Input: part model. Units: mm. Frame: model coordinates. Face numbers are marked on the shaded views. Coordinates: 2 decimals unless noted, no trailing zeros. Order: outer loops, then holes, each group sorted by start corner. A loop starts at its lowest first (then second) coordinate and runs counter-clockwise, first axis right, second up. Notation, with made-up numbers: (-23.75, 12) -> (28.25, 12) arc R15 cw to (28.25, 17) -> close; hole circle Ø4 at (52.5, -34). An arc over 180 degrees is marked (long way). One line per question, with ' | ' between items.
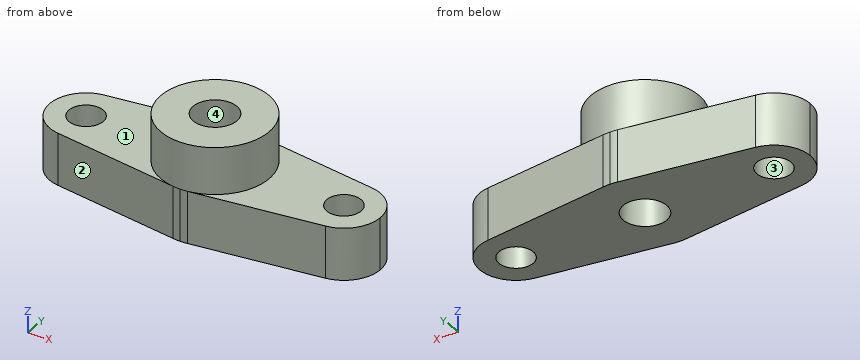
```python
from build123d import *

# Parameters (mm, degrees)
SKETCH_1_W             = 32
SKETCH_1_H             = 10.4
SKETCH_1_R             = 0.5
EXTRUDE_1_DEPTH        = 5
SKETCH_2_R             = 5.2
SKETCH_2_R_2           = 0.5
EXTRUDE_2_DEPTH        = 4.5
CUT_EXTRUDE_START      = -5.3
CUT_EXTRUDE_1_DEPTH    = 5.3
HOLE_WIZARD_M4_1_D     = 3.3
HOLE_WIZARD_M4_1_DEPTH = 10.1
HOLE_WIZARD_M4_1_TIP   = 0.991420021
HOLE_WIZARD_M5_1_D     = 4.2
HOLE_WIZARD_M5_1_DEPTH = 22.4
HOLE_WIZARD_M5_1_TIP   = 1.2618073


with BuildPart() as part:
    # 草图1 → 凸台-拉伸1 (new body)
    with BuildSketch(Plane.XY):
        Rectangle(SKETCH_1_W, SKETCH_1_H)
        with Locations((-12.5, 0)):
            Circle(SKETCH_1_R, mode=Mode.SUBTRACT)
        with Locations((12.5, 0)):
            Circle(SKETCH_1_R, mode=Mode.SUBTRACT)
        Circle(SKETCH_1_R, mode=Mode.SUBTRACT)
    extrude(amount=EXTRUDE_1_DEPTH)

    # 草图2 → 凸台-拉伸2 (add)
    with BuildSketch(Plane.XY.offset(5)):
        with Locations(Location((0, 0, 0), (0, 0, 270))):
            Circle(SKETCH_2_R)
        Circle(SKETCH_2_R_2, mode=Mode.SUBTRACT)
    extrude(amount=EXTRUDE_2_DEPTH)

    # 草图3 → 切除-拉伸1 (cut)
    with BuildSketch(Plane.XY.offset(5).offset(CUT_EXTRUDE_START)):
        with BuildLine():
            Line((-12.976, 3.46748093), (-0.7072, 5.151685953))
            ThreePointArc((-0.7072, 5.151685953), (-0.354424212, 5.187907428), (0, 5.2))
            Line((0, 5.2), (-16, 5.2))
            Line((-16, 5.2), (-16, 0))
            ThreePointArc((-16, 0), (-15.137802115, 2.300434742), (-12.976, 3.46748093))
        make_face()
        with BuildLine():
            ThreePointArc((0, -5.2), (-0.354424212, -5.187907428), (-0.7072, -5.151685953))
            Line((-0.7072, -5.151685953), (-12.976, -3.46748093))
            ThreePointArc((-12.976, -3.46748093), (-15.137802115, -2.300434742), (-16, 0))
            Line((-16, 0), (-16, -5.2))
            Line((-16, -5.2), (0, -5.2))
        make_face()
        with BuildLine():
            ThreePointArc((0.7072, -5.151685953), (0.354424212, -5.187907428), (0, -5.2))
            Line((0, -5.2), (16, -5.2))
            Line((16, -5.2), (16, 0))
            ThreePointArc((16, 0), (15.137802115, -2.300434742), (12.976, -3.46748093))
            Line((12.976, -3.46748093), (0.7072, -5.151685953))
        make_face()
        with BuildLine():
            Line((16, 5.2), (0, 5.2))
            ThreePointArc((0, 5.2), (0.354424212, 5.187907428), (0.7072, 5.151685953))
            Line((0.7072, 5.151685953), (12.976, 3.46748093))
            ThreePointArc((12.976, 3.46748093), (15.137802115, 2.300434742), (16, 0))
            Line((16, 0), (16, 5.2))
        make_face()
    extrude(amount=CUT_EXTRUDE_1_DEPTH, mode=Mode.SUBTRACT)

    # M4 螺纹孔1
    with Locations(Plane.XY.offset(5)):
        with Locations((-12.5, 0), (12.5, 0)):
            Hole(HOLE_WIZARD_M4_1_D / 2, depth=HOLE_WIZARD_M4_1_DEPTH)
            with Locations((0, 0, -(HOLE_WIZARD_M4_1_DEPTH + HOLE_WIZARD_M4_1_TIP / 2))):  # 118° drill point
                Cone(0, HOLE_WIZARD_M4_1_D / 2, HOLE_WIZARD_M4_1_TIP, mode=Mode.SUBTRACT)

    # M5 螺纹孔1
    with Locations(Plane.XY.offset(9.5)):
        with Locations((0, 0)):
            Hole(HOLE_WIZARD_M5_1_D / 2, depth=HOLE_WIZARD_M5_1_DEPTH)
            with Locations((0, 0, -(HOLE_WIZARD_M5_1_DEPTH + HOLE_WIZARD_M5_1_TIP / 2))):  # 118° drill point
                Cone(0, HOLE_WIZARD_M5_1_D / 2, HOLE_WIZARD_M5_1_TIP, mode=Mode.SUBTRACT)


solid = part.part
```
1. Ray query, line 1 (Y direction, x = 0, z = 4.5); line 2 (X direction, y = -0.75, z = 1); line 3 (Z direction, x = -7.5, y = -3.25). Return the intervals inside material, ascending. Write a range as [from, to].
Recorded:
line 1: y = [-5.2, -2.1], [2.1, 5.2] | line 2: x = [-15.92, -13.97], [-11.03, -1.96], [1.96, 11.03], [13.97, 15.92] | line 3: z = [0, 5]
2. Cut plane A-A, the plane z = 1. Return loops of the section in (x, y).
Recorded:
outline: (-12.98, -3.47) -> (-0.71, -5.15) arc R5.2 ccw to (0.71, -5.15) -> (12.98, -3.47) arc R3.5 ccw to (12.98, 3.47) -> (0.71, 5.15) arc R5.2 ccw to (-0.71, 5.15) -> (-12.98, 3.47) arc R3.5 ccw to start; hole circle Ø3.3 at (-12.5, 0); hole circle Ø4.2 at (0, 0); hole circle Ø3.3 at (12.5, 0)
3. Cut plane B-B, the plane x = 12.5. Return loops of the section in (y, z).
Recorded:
outline: (-3.53, 0) -> (-1.65, 0) -> (-1.65, 5) -> (-3.53, 5) -> close; (1.65, 0) -> (3.53, 0) -> (3.53, 5) -> (1.65, 5) -> close
4. Pin query (flat end, axial travel): pin 1 Ø4.5 at (x, y) = (12.5, 0) entering from +Z; pin 2 Ø3 at (x, y) = (-12.5, 0) entering from -Z. Return the tip coordinate at first contact, or that it passes through.
Recorded:
pin 1: stops at z = 5 | pin 2: passes through
5. Cut plane C-C, the plane z = 7. Return loops of the section in (x, y), and give its area (3 significant figures).
Recorded:
outline: circle Ø10.4 at (0, 0); hole circle Ø4.2 at (0, 0) | area: 71.1 mm^2
6. Cut plane D-D, the plane y = -2.5. Return loops of the section in (x, z).
Recorded:
outline: (-14.95, 0) -> (14.95, 0) -> (14.95, 5) -> (4.56, 5) -> (4.56, 9.5) -> (-4.56, 9.5) -> (-4.56, 5) -> (-14.95, 5) -> close
7. Mould query, pull axis Y, two halves, no side actions, for the marked faces 1, 2, 3 and 4. Classes: released by +Y, released by -Y, zero draft, split by the parting line, or undercut.
Recorded:
face 1: zero draft | face 2: released by -Y | face 3: undercut | face 4: undercut
